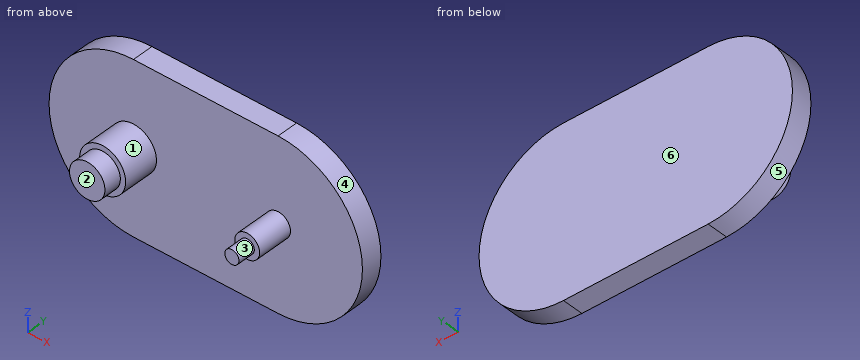
from build123d import *

# Parameters (mm, degrees)
BOSS_EXTRU_1_DEPTH = 3
ESQUISSE2_R        = 3.25
ESQUISSE2_R_2      = 1.75
BOSS_EXTRU_2_DEPTH = 5
ESQUISSE3_R        = 2.5
ESQUISSE3_R_2      = 1
BOSS_EXTRU_3_DEPTH = 2.5


with BuildPart() as part:
    # Esquisse1 → Boss.-Extru.1 (new body)
    with BuildSketch(Plane(origin=(0, 0, 0), x_dir=(1, 0, 0), z_dir=(0, 1, 0))):
        with BuildLine():
            Line((10.2, -11.9), (-10.2, -11.9))
            ThreePointArc((-10.2, -11.9), (-22.1, 0), (-10.2, 11.9))
            Line((-10.2, 11.9), (10.2, 11.9))
            ThreePointArc((10.2, 11.9), (22.1, 0), (10.2, -11.9))
        make_face()
    extrude(amount=BOSS_EXTRU_1_DEPTH)

    # Esquisse2 → Boss.-Extru.2 (add)
    with BuildSketch(Plane.XZ):
        with Locations(Location((-10.2, 0, 0), (0, 0, 90))):
            Circle(ESQUISSE2_R)
        with Locations(Location((10.2, 0, 0), (0, 0, 90))):
            Circle(ESQUISSE2_R_2)
    extrude(amount=BOSS_EXTRU_2_DEPTH)

    # Esquisse3 → Boss.-Extru.3 (add)
    with BuildSketch(Plane.XZ.offset(5)):
        with Locations(Location((-10.2, 0, 0), (0, 0, 270))):
            Circle(ESQUISSE3_R)
        with Locations(Location((10.2, 0, 0), (0, 0, 270))):
            Circle(ESQUISSE3_R_2)
    extrude(amount=BOSS_EXTRU_3_DEPTH)


solid = part.part
Work out the finished part from the listing and answer in its coordinate system (mm). Face numbers are marked on the shaded views. A direction names the side the tool comes from. Round coordinates to 2 decimals unless told otherwise and drop trailing zeros. Loops run counter-clockwise (first coordinate to the right, second up) from the corner with the lowest first, then second, coordinate; pieces in that order, holes last. Notation, with made-up numbers: (15.5, -9.5) - (42.5, -9.5) arc R21 cw to (42.5, 27.5) - close; hole circle Ø5 at (4.25, -33.75). An arc over 180 degrees is marked (long way). Use one line per item in the form item = value. Start each with the question number.
(1) Find section C-C on x = -0.5. Determine the outline of the cut face in (y, z), and give its area (3 significant figures).
(2) Which of the six approach directions +Z, -Z, +X, -X, +Y, -Y give full straight-line access (tool end or side, diameter ignored) to the marked faces 1 and 2?
(3) Find section A-A on z = 0. Determine the outline of the cut face in (x, y).
(4) Determine the mould class of the marked faces 3, 4, 5 and 6 for opening direction X: +X half, -X half, draft (parallel to the pull), parting line (faces both ways), or undercut.
(5) Flat-ended cylindrical pins translate along their axes: P1, Ø1.5, axis at y = -0.5, z = -5.5, coming from the +X side; P2, Ø5, axis at y = -5.5, z = -4.5, coming from the -X side; P3, Ø1, axis at x = -16, y = 0, coming from the +Z side. Find the tip coordinate at first contact, or state that the pin passes through.
(6) Find section B-B on y = -4.5. Determine the outline of the cut face in (x, z).
(7) Consider line 1 (Y direction, x = -15, z = 3); line 2 (X direction, y = 2.25, z = 0.5); line 3 (X direction, y = 2.5, z = 10.5). Determine where each line is inside the solid, lowest interval first.
(8) Find section D-D on y = 1.5. Determine the outline of the cut face in (x, z).
Answer list:
q1.outline = (0, -11.9) - (3, -11.9) - (3, 11.9) - (0, 11.9) - close
q1.area = 71.4 mm^2
q2.face_1 = -Y
q2.face_2 = +Z, -Z, +X, -X, -Y
q3.outline = (-22.1, 0) - (-13.45, 0) - (-13.45, -5) - (-12.7, -5) - (-12.7, -7.5) - (-7.7, -7.5) - (-7.7, -5) - (-6.95, -5) - (-6.95, 0) - (8.45, 0) - (8.45, -5) - (9.2, -5) - (9.2, -7.5) - (11.2, -7.5) - (11.2, -5) - (11.95, -5) - (11.95, 0) - (22.1, 0) - (22.1, 3) - (-22.1, 3) - close
q4.face_3 = undercut
q4.face_4 = +X half
q4.face_5 = -X half
q4.face_6 = draft
q5.P1 = 21.03
q5.P2 = -12.72
q5.P3 = 10.65
q6.outline = circle Ø6.5 at (-10.2, 0); circle Ø3.5 at (10.2, 0)
q7.line_1 = 0 to 3
q7.line_2 = -22.09 to 22.09
q7.line_3 = -15.8 to 15.8
q8.outline = (-10.2, -11.9) - (10.2, -11.9) arc R11.9 ccw to (10.2, 11.9) - (-10.2, 11.9) arc R11.9 ccw to start
